Geometry check sheet. Reference: drawing and pictorial views, mm from the part's lowest x, y, z. A direction names the side the tool comes from. Coordinates: 2 decimals unless noted, no trailing zeros. Write each loop counter-clockwise with the first axis right and the second up, starting at its lowest first coordinate (ties: lowest second). Pieces come first, ordered by that corner, then holes. Notation, with made-up numbers: (-38.5, 52) -> (-18.5, 52) arc R15 ccw to (-18.5, 81) -> close; hole circle Ø5 at (-1.75, 60.5). An arc over 180 degrees is marked (long way). Put each result on its own line as item: value.
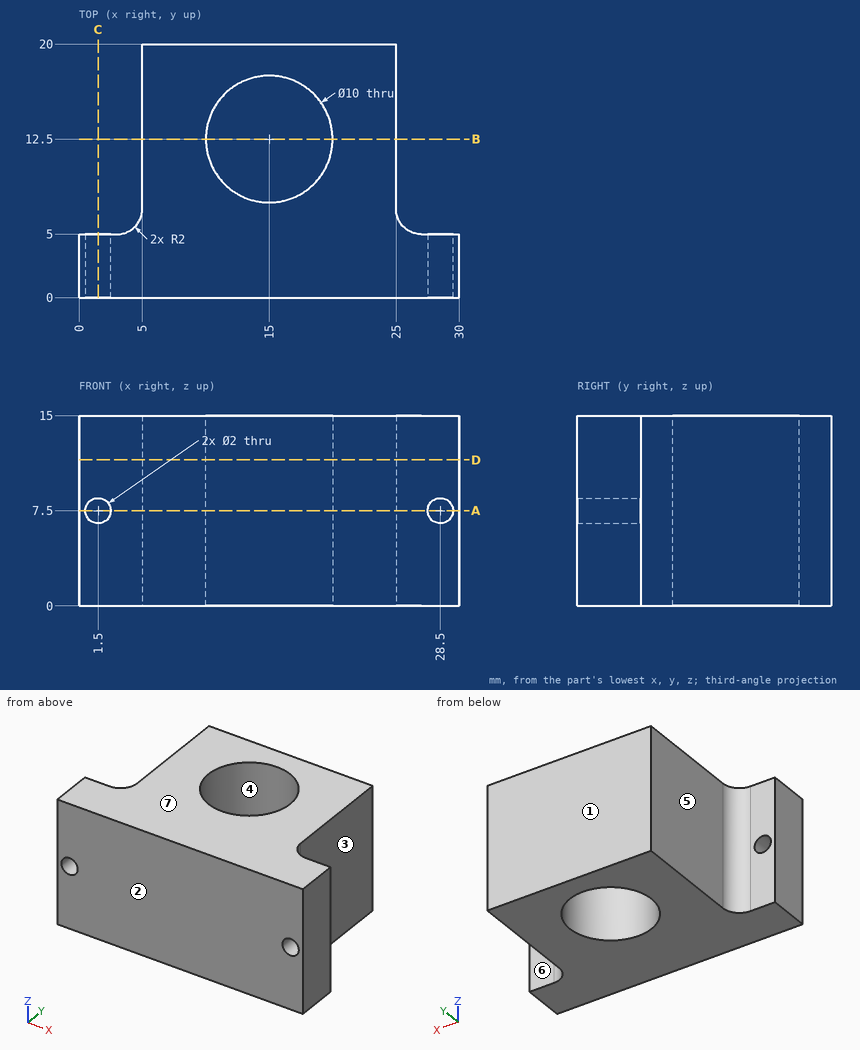
Q1. Cross-section at D-D (z = 11.5). Record the cut outline in (x, y), plus the area to 3 significant figures.
Recorded:
outline: (0, 0) -> (30, 0) -> (30, 5) -> (27, 5) arc R2 cw to (25, 7) -> (25, 20) -> (5, 20) -> (5, 7) arc R2 cw to (3, 5) -> (0, 5) -> close; hole circle Ø10 at (15, 12.5)
area: 373 mm2
Q2. Material ranges on line 1 along Z through (x, y) = (1.5, 3.3); line 2 along Y through (x, z) = (14.75, 8.5); line 3 along X through (y, z) = (18.25, 12.75), recorded low to high.
Recorded:
line 1: z = 0 to 6.5, 8.5 to 15
line 2: y = 0 to 7.51, 17.49 to 20
line 3: x = 5 to 25
Q3. Tool access check on the marked faces 5, 6 and 7. Record the directions out of +Z, -Z, +X, -X, +Y, -Y that give a thin tool (end or side, any length) a straight path to the whole face; none if there is none.
Recorded:
face 5: +Z, -Z, -X, +Y
face 6: +Z, -Z, +X, +Y
face 7: +Z, +X, -X, +Y, -Y
Q4. Cross-section at C-C (x = 1.5). Record the cut outline in (y, z), plus the area to 3 significant figures.
Recorded:
outline: (0, 0) -> (5, 0) -> (5, 6.5) -> (0, 6.5) -> close; (0, 8.5) -> (5, 8.5) -> (5, 15) -> (0, 15) -> close
area: 65.0 mm2
Q5. Cross-section at A-A (z = 7.5). Record the cut outline in (x, y), plus the area to 3 significant figures.
Recorded:
outline: (0, 0) -> (0.5, 0) -> (0.5, 5) -> (0, 5) -> close; (2.5, 0) -> (27.5, 0) -> (27.5, 5) -> (27, 5) arc R2 cw to (25, 7) -> (25, 20) -> (5, 20) -> (5, 7) arc R2 cw to (3, 5) -> (2.5, 5) -> close; (29.5, 0) -> (30, 0) -> (30, 5) -> (29.5, 5) -> close; hole circle Ø10 at (15, 12.5)
area: 353 mm2
Q6. Depth check by flat-ended pin: P1, Ø9, axis at x = 15, y = 12.5, coming from the +Z side; P2, Ø4, axis at y = 12.5, z = 5.5, coming from the -X side; P3, Ø3.5, axis at x = 2, z = 6, coming from the +Y side; P4, Ø6, axis at y = 18, z = 4, coming from the +X side. Enter the tip coordinate at first touch or a pass-through.
Recorded:
P1: passes through
P2: stops at x = 5
P3: stops at y = 5.15
P4: stops at x = 25
Q7. Cross-section at B-B (y = 12.5). Record the cut outline in (x, z).
Recorded:
outline: (5, 0) -> (10, 0) -> (10, 15) -> (5, 15) -> close; (20, 0) -> (25, 0) -> (25, 15) -> (20, 15) -> close
Q8. Mould release check, pull along Y, two halves, no side actions. Record for the marked faces 1, 2, 3 and 4: released by +Y, released by -Y, zero draft, split by the parting line, or undercut.
Recorded:
face 1: released by +Y
face 2: released by -Y
face 3: zero draft
face 4: undercut
